Check sheet for the drawn part. Datum: minimum x, y, z corner. Units: mm. A direction names the side the tool comes from. Round coordinates to 2 decimals unless told otherwise and drop trailing zeros. Write each loop counter-clockwise with the first axis right and the second up, starting at its lowest first coordinate (ties: lowest second). Pieces come first, ordered by that corner, then holes. Notation, with made-up numbers: M 19,72.5 L 75,72.5 A14 cw 75,79.5 Z; hole C -11,34.5 d8. An arc over 180 degrees is marked long. Use a Markdown table: item, result.
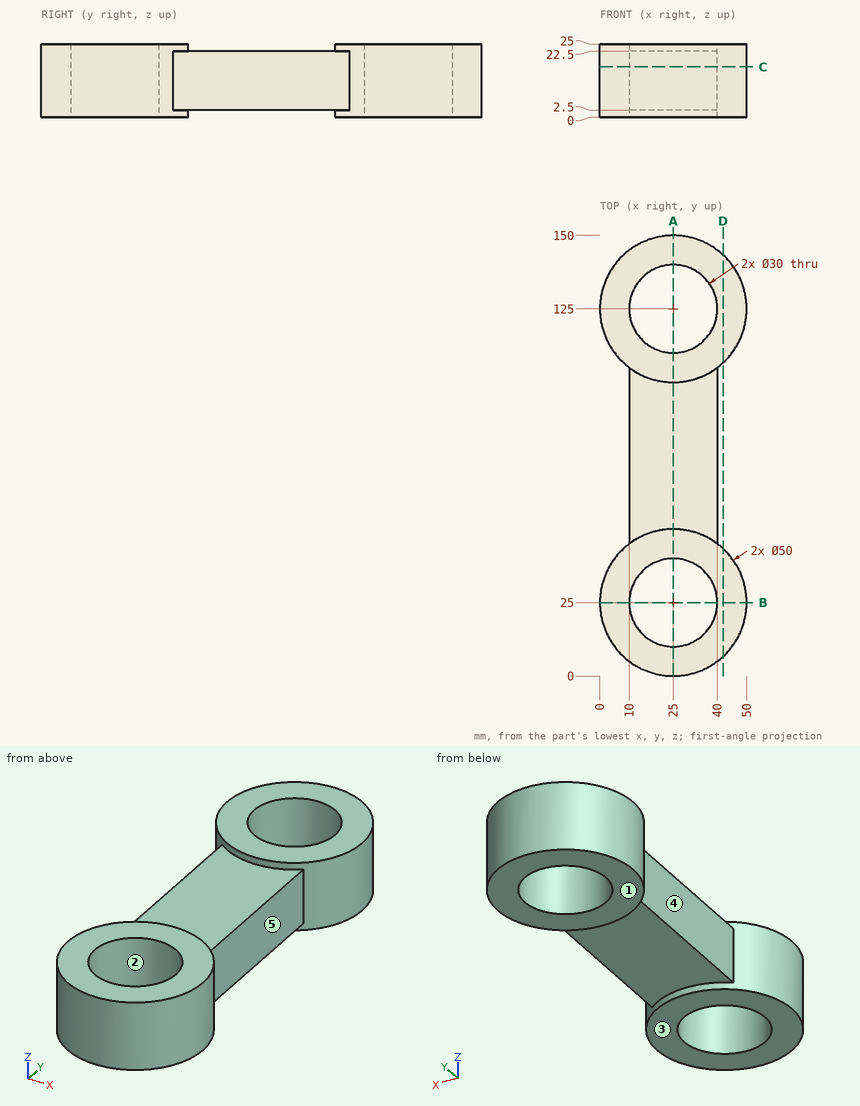
Item 1: Cross-section at A-A, the plane x = 25. Record the cut outline in (y, z), and give its area (3 significant figures).
Outcome:
| item | result |
|---|---|
| outline | M 0,0 L 10,0 L 10,25 L 0,25 Z; M 40,0 L 50,0 L 50,2.5 L 100,2.5 L 100,0 L 110,0 L 110,25 L 100,25 L 100,22.5 L 50,22.5 L 50,25 L 40,25 Z; M 140,0 L 150,0 L 150,25 L 140,25 Z |
| area | 2,000 mm2 |
Item 2: Go/stop test with flat-tipped pins: pin 1 (5 mm diameter, centred on x = 38.5, y = 94, fed in from +Z); pin 2 (1.5 mm diameter, centred on y = 100, z = 10, fed in from +X); pin 3 (12 mm diameter, centred on x = 13, z = 17, fed in from -Y); pin 4 (24 mm diameter, centred on x = 25, y = 125, fed in from -Z). Record where each tip stops, or that it passes through.
Outcome:
| item | result |
|---|---|
| pin 1 | stops at z = 22.5 |
| pin 2 | stops at x = 40 |
| pin 3 | stops at y = 0.73 |
| pin 4 | passes through |
Item 3: Cross-section at C-C, the plane z = 17.25. Record the cut outline in (x, y), and give its area (3 significant figures).
Outcome:
| item | result |
|---|---|
| outline | M 10,45 A25 ccw long 40,45 L 40,105 A25 ccw long 10,105 Z; hole C 25,25 d30; hole C 25,125 d30 |
| area | 4,110 mm2 |
Item 4: Mould release check, pull along Y, two halves, no side actions. Record for the marked faces 1 and 2: +Y half, -Y half, draft (parallel to the pull), parting line (faces both ways), or undercut.
Outcome:
| item | result |
|---|---|
| face 1 | draft |
| face 2 | undercut |
Item 5: Material ranges on line 1 along Y through (x, z) = (25, 12.25); line 2 along Z through (x, y) = (34, 94); line 3 along X through (y, z) = (95.5, 9), recorded low to high. Write a range as from..to.
Outcome:
| item | result |
|---|---|
| line 1 | y = 0..10, 40..110, 140..150 |
| line 2 | z = 2.5..22.5 |
| line 3 | x = 10..40 |
Item 6: Access from +Z, -Z, +X, -X, +Y, -Y to the whole of each face (thin tool, end or side, straight path). Record for the marked faces 3, 4 and 5.
Outcome:
| item | result |
|---|---|
| face 3 | -Z, +X, -X, +Y, -Y |
| face 4 | +Z, -Z, -X |
| face 5 | +Z, -Z, +X |
Item 7: Cross-section at B-B, the plane y = 25. Record the cut outline in (x, z), and give its area (3 significant figures).
Outcome:
| item | result |
|---|---|
| outline | M 0,0 L 10,0 L 10,25 L 0,25 Z; M 40,0 L 50,0 L 50,25 L 40,25 Z |
| area | 500 mm2 |
Item 8: Cross-section at D-D, the plane x = 42. Record the cut outline in (y, z).
Outcome:
| item | result |
|---|---|
| outline | M 6.67,0 L 43.33,0 L 43.33,25 L 6.67,25 Z; M 106.67,0 L 143.33,0 L 143.33,25 L 106.67,25 Z |
